Can you work these out from the model? Positions are in its coordinate system, mm. Face numbers are marked on the shaded views. Coordinates: 2 decimals unless noted, no trailing zeros. Order: outer loops, then holes, each group sorted by start corner. A loop starts at its lowest first (then second) coordinate and runs counter-clockwise, first axis right, second up. Notation, with made-up numbers: (73.25, -29) -> (117.25, -29) arc R17 cw to (117.25, -15) -> close; hole circle Ø7 at (-35, 26.5). An arc over 180 degrees is marked (long way). Answer in a Markdown table with one row per item. Add a question column.
1. If I drill on line 1 along Y through (x, z) = (-5.1, -4.9) (3 decimals); line 2 along Z through (x, y) = (-2.5, 54); line 3 along Y through (x, z) = (-0.25, 1.5), over which ranges is the centre line in solid material (lowest first)? Write a range as [from, to].
2. We'd pull the mould along Y, two halves only. Please class the marked faces 1 and 2: pulls with the +Y half, pulls with the -Y half, needs draft (parallel to the pull), parting line crosses it, or undercut.
3. Imagine slicing it at C-C on z = 44. Write out the boundary of the cut face in (x, y).
4. Imagine slicing it at A-A on z = -4.9. Write out the boundary of the cut face in (x, y) (3 decimals).
5. Will these pins go through, and if not, where does the flat tip stop? pin 1 (3 mm diameter, centred on y = 83.125, z = -4.9, fed in from +X); pin 2 (12 mm diameter, centred on y = 67, z = 23, fed in from -X); pin 3 (1.7 mm diameter, centred on x = -1.5, z = 17.5, fed in from -Y); pin 4 (2.5 mm diameter, centred on x = -8.5, z = 26, fed in from +Y).
from build123d import *
from OCP.BRepFilletAPI import BRepFilletAPI_MakeChamfer

# Parameters (mm, degrees)
SKETCH2_W           = 95
SKETCH2_H           = 50
BOSS_EXTRUDE1_DEPTH = 10
SKETCH3_W           = 3.3
SKETCH3_H           = 9.8
BOSS_EXTRUDE2_DEPTH = 95
SKETCH4_W           = 3.3
SKETCH4_H           = 59.8
BOSS_EXTRUDE3_DEPTH = 4.9
CUT_EXTRUDE1_REACH  = 113.912
SKETCH5_R           = 1.9
LPATTERN1_COUNT     = 4
LPATTERN1_PITCH     = 23.75
SKETCH7_W           = 3.5
SKETCH7_H           = 104.8
CUT_EXTRUDE6_DEPTH  = 5
SKETCH8_W           = 85
SKETCH8_H           = 35
CUT_EXTRUDE7_DEPTH  = 5
CHAMFER1_SIZE       = 2.5
CHAMFER1_SIZE_2     = 5


with BuildPart() as part:
    # Sketch2 → Boss-Extrude1 (new body)
    with BuildSketch(Plane.YZ):
        with Locations((47.5, 25)):
            Rectangle(SKETCH2_W, SKETCH2_H)
    extrude(amount=-BOSS_EXTRUDE1_DEPTH)

    # Sketch3 → Boss-Extrude2 (add)
    with BuildSketch(Plane(origin=(0, 95, 0), x_dir=(-1, 0, 0), z_dir=(0, 1, 0))):
        with Locations((5, -4.9)):
            Rectangle(SKETCH3_W, SKETCH3_H)
    extrude(amount=-BOSS_EXTRUDE2_DEPTH)

    # Sketch4 → Boss-Extrude3 (add)
    with BuildSketch(Plane(origin=(0, 95, 0), x_dir=(-1, 0, 0), z_dir=(0, 1, 0))):
        with Locations((5, 20.1)):
            Rectangle(SKETCH4_W, SKETCH4_H)
    boss_extrude3 = extrude(amount=BOSS_EXTRUDE3_DEPTH)

    # Mirror1: Boss-Extrude3 across plane
    add(boss_extrude3.mirror(Plane.ZX.offset(47.5)))

    # Sketch5 → Cut-Extrude1 (cut, up to next)
    with BuildSketch(Plane.YZ.offset(-3.35), mode=Mode.PRIVATE) as cut_extrude1_sk1:
        with Locations(Location((11.875, -4.9, 0), (0, 0, 270))):
            Circle(SKETCH5_R)
    cut_extrude1_tool1 = extrude(cut_extrude1_sk1.sketch, amount=-CUT_EXTRUDE1_REACH, mode=Mode.PRIVATE) & part.part
    cut_extrude1 = cut_extrude1_tool1.solids().sort_by_distance((-3.35, 11.875, -4.9))[0]
    add(cut_extrude1, mode=Mode.SUBTRACT)

    # LPattern1: Cut-Extrude1 ×4
    with Locations(*[(0, i * LPATTERN1_PITCH, 0) for i in range(1, LPATTERN1_COUNT)]):
        add(cut_extrude1, mode=Mode.SUBTRACT)

    # Sketch7 → Cut-Extrude6 (cut)
    with BuildSketch(Plane.XY.offset(50)):
        with Locations((-5, 47.5)):
            Rectangle(SKETCH7_W, SKETCH7_H)
    extrude(amount=-CUT_EXTRUDE6_DEPTH, mode=Mode.SUBTRACT)

    # Sketch8 → Cut-Extrude7 (cut)
    with BuildSketch(Plane(origin=(-10, 0, 0), x_dir=(0, -1, 0), z_dir=(-1, 0, 0))):
        with Locations((-47.5, 22.5)):
            Rectangle(SKETCH8_W, SKETCH8_H)
    extrude(amount=-CUT_EXTRUDE7_DEPTH, mode=Mode.SUBTRACT)

    # Chamfer1
    chamfer1_edges_1 = [part.edges().sort_by_distance(p)[0] for p in [
        (-10, 5, 22.5),
    ]]
    chamfer1_side_1 = [part.faces().sort_by_distance(p)[0] for p in [
        (-10, 4.95, 22.5),
    ]]
    chamfer1_edges_2 = [part.edges().sort_by_distance(p)[0] for p in [
        (-10, 47.5, 5),
    ]]
    chamfer1_side_2 = [part.faces().sort_by_distance(p)[0] for p in [
        (-10, 47.5, 4.95),
    ]]
    chamfer1_edges_3 = [part.edges().sort_by_distance(p)[0] for p in [
        (-10, 90, 22.5),
    ]]
    chamfer1_side_3 = [part.faces().sort_by_distance(p)[0] for p in [
        (-10, 90.05, 22.5),
    ]]
    chamfer1_edges_4 = [part.edges().sort_by_distance(p)[0] for p in [
        (-10, 47.5, 40),
    ]]
    chamfer1_side_4 = [part.faces().sort_by_distance(p)[0] for p in [
        (-10, 47.5, 40.05),
    ]]
    chamfer1 = BRepFilletAPI_MakeChamfer(part.part.solid().wrapped)
    for e in chamfer1_edges_1:
        chamfer1.Add(CHAMFER1_SIZE - 0.0001, CHAMFER1_SIZE_2 - 0.0001, e.wrapped, chamfer1_side_1[0].wrapped)
    for e in chamfer1_edges_2:
        chamfer1.Add(CHAMFER1_SIZE - 0.0001, CHAMFER1_SIZE_2 - 0.0001, e.wrapped, chamfer1_side_2[0].wrapped)
    for e in chamfer1_edges_3:
        chamfer1.Add(CHAMFER1_SIZE - 0.0001, CHAMFER1_SIZE_2 - 0.0001, e.wrapped, chamfer1_side_3[0].wrapped)
    for e in chamfer1_edges_4:
        chamfer1.Add(CHAMFER1_SIZE - 0.0001, CHAMFER1_SIZE_2 - 0.0001, e.wrapped, chamfer1_side_4[0].wrapped)
    add(Compound.cast(chamfer1.Shape()), mode=Mode.REPLACE)  # a hair under: the kernel refuses the full size


solid = part.part
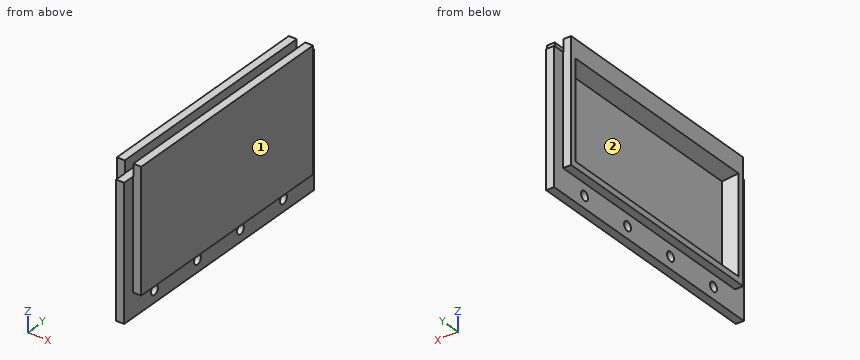
Answers follow:
| question | item | result |
|---|---|---|
| 1 | line 1 | y = [-4.9, 9.975], [13.775, 33.725], [37.525, 57.475], [61.275, 81.225], [85.025, 99.9] |
| 1 | line 2 | z = [0, 50] |
| 1 | line 3 | y = [0, 95] |
| 2 | face 1 | needs draft |
| 2 | face 2 | undercut |
| 3 | outline | (-10, 0) -> (-6.65, 0) -> (-6.65, -4.9) -> (-3.35, -4.9) -> (-3.35, 0) -> (0, 0) -> (0, 95) -> (-3.35, 95) -> (-3.35, 99.9) -> (-6.65, 99.9) -> (-6.65, 95) -> (-10, 95) -> close |
| 4 | outline | (-6.65, -4.9) -> (-3.35, -4.9) -> (-3.35, 9.975) -> (-6.65, 9.975) -> close; (-6.65, 13.775) -> (-3.35, 13.775) -> (-3.35, 33.725) -> (-6.65, 33.725) -> close; (-6.65, 37.525) -> (-3.35, 37.525) -> (-3.35, 57.475) -> (-6.65, 57.475) -> close; (-6.65, 61.275) -> (-3.35, 61.275) -> (-3.35, 81.225) -> (-6.65, 81.225) -> close; (-6.65, 85.025) -> (-3.35, 85.025) -> (-3.35, 99.9) -> (-6.65, 99.9) -> close |
| 5 | pin 1 | passes through |
| 5 | pin 2 | stops at x = -5 |
| 5 | pin 3 | stops at y = 0 |
| 5 | pin 4 | stops at y = 95 |
